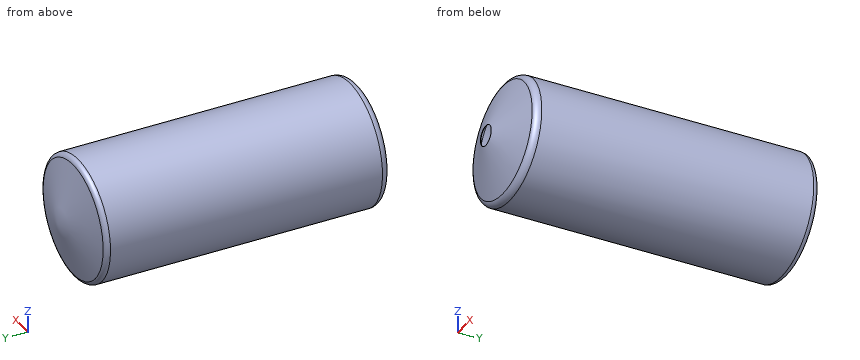
```python
from build123d import *


with BuildPart() as part:
    # Skizze1 → Rotation4 (revolve)
    with BuildSketch(Plane.XY, mode=Mode.PRIVATE) as rotation4_sk:
        with BuildLine():
            Line((-75, 27.29776757), (-413.811107883, 150.614925878))
            ThreePointArc((-413.811107883, 150.614925878), (-440.053362436, 170.751316022), (-450, 202.298020021))
            Line((-450, 202.298020021), (-450, 2202.298020021))
            ThreePointArc((-450, 2202.298020021), (-441.734133612, 2226.648477182), (-420.352761804, 2240.935053073))
            Line((-420.352761804, 2240.935053073), (0, 2353.568236134))
            Line((0, 2353.568236134), (0, 2350.980045683))
            Line((0, 2350.980045683), (-419.705714191, 2238.520238507))
            ThreePointArc((-419.705714191, 2238.520238507), (-439.750750261, 2225.126573609), (-447.5, 2202.298020021))
            Line((-447.5, 2202.298020021), (-447.5, 202.298020021))
            ThreePointArc((-447.5, 202.298020021), (-438.005482325, 172.185257113), (-412.956057525, 152.96415743))
            Line((-412.956057525, 152.96415743), (-75, 29.958212001))
            Line((-75, 29.958212001), (-75, 27.29776757))
        make_face()
    revolve(rotation4_sk.sketch.rotate(Axis((0, 0, 0), (0, 1, 0)), 270), axis=Axis((0, 0, 0), (0, 1, 0)))  # turned: the seam where the file's is


solid = part.part
```
The model under review builds one solid part; all positions refer to its coordinate system, in mm. Round coordinates to 2 decimals unless told otherwise and drop trailing zeros. Loops run counter-clockwise (first coordinate to the right, second up) from the corner with the lowest first, then second, coordinate; pieces in that order, holes last. Notation, with made-up numbers: (34, -37.75) - (68, -37.75) arc R15 cw to (68, -16.75) - close; hole circle Ø7 at (-5, 73). An arc over 180 degrees is marked (long way). Write each question's results on one line, items separated by ' | '. Start each with the question number.
Q1. Insertion check: P1, Ø4, axis at x = 173, y = 845.5, coming from the +Z side; P2, Ø4, axis at x = 114, z = 121.5, coming from the +Y side; P3, Ø5, axis at x = 241.5, z = 16, coming from the +Y side. Each pin has a flat end and moves straight along its axis. Give the tip position at first contact, or say it passes through.
Q2. Wall thickness on line 1 along X through (y, z) = (1233, 0); line 2 along X through (y, z) = (2050, -90.5); line 3 along Y through (x, z) = (387.5, 206): over which ranges is each line inside the solid? List them lowest first. Write a range as [from, to].
Q3. Take a section at A-A on y = 2126.5. Give the boundary of the cut face in (x, z).
Data:
1) P1: stops at z = 416.24 | P2: stops at y = 2309.46 | P3: stops at y = 2289.39
2) line 1: x = [-450, -447.5], [447.5, 450] | line 2: x = [-440.81, -438.25], [438.25, 440.81] | line 3: y = [169.1, 173.43], [2226.25, 2230]
3) outline: circle Ø900 at (0, 0); hole circle Ø895 at (0, 0)
